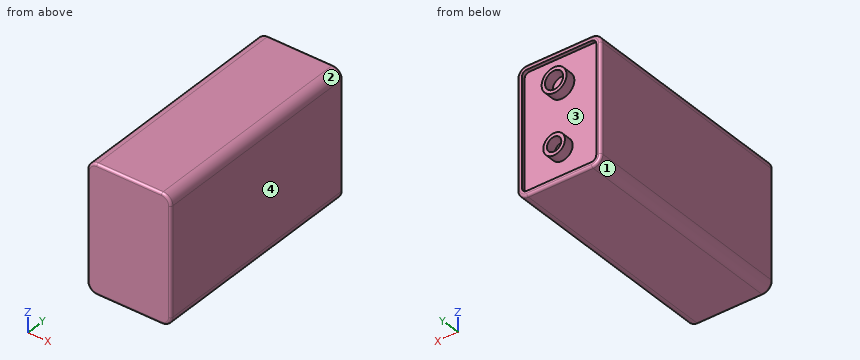
Autodesk Fusion 360 part; units mm, degrees
sketch "Sketch1" plane through (0, 0, 0) normal (0, 1, 0) x (1, 0, 0)
  line L0 (6.75, 13.25) -> (-6.75, 13.25)
  line L1 (-8.75, 11.25) -> (-8.75, -11.25)
  line L2 (-6.75, -13.25) -> (6.75, -13.25)
  line L3 (8.75, -11.25) -> (8.75, 11.25)
  arc A0 (-6.75, 13.25) -> (-8.75, 11.25) centre (-6.75, 11.25) ccw
  arc A1 (8.75, 11.25) -> (6.75, 13.25) centre (6.75, 11.25) ccw
  arc A2 (6.75, -13.25) -> (8.75, -11.25) centre (6.75, -11.25) ccw
  arc A3 (-8.75, -11.25) -> (-6.75, -13.25) centre (-6.75, -11.25) ccw
  point P0 (8.75, 13.25)
  point P1 (-8.75, 13.25)
  point P2 (8.75, -13.25)
  dimension "d1" = 17.5
  dimension "d2" = 26.5
  dimension "d3" = 2
extrude "Extrude1" add sketch "Sketch1" along normal blind 46.4
sketch "Sketch2" plane through (0, 46.4, 0) normal (0, 1, 0) x (-1, 0, 0)
  arc A0 (8.75, 11.25) -> (6.75, 13.25) centre (6.75, 11.25) ccw
  line L0 (6.75, 13.25) -> (-6.75, 13.25)
  arc A1 (-6.75, 13.25) -> (-8.75, 11.25) centre (-6.75, 11.25) ccw
  line L1 (-8.75, 11.25) -> (-8.75, -11.25)
  arc A2 (-8.75, -11.25) -> (-6.75, -13.25) centre (-6.75, -11.25) ccw
  line L2 (-6.75, -13.25) -> (6.75, -13.25)
  arc A3 (6.75, -13.25) -> (8.75, -11.25) centre (6.75, -11.25) ccw
  line L3 (8.75, -11.25) -> (8.75, 11.25)
  line L4 (7.75, -11.25) -> (7.75, 11.25)
  arc A4 (7.75, 11.25) -> (6.75, 12.25) centre (6.75, 11.25) ccw
  line L5 (6.75, 12.25) -> (-6.75, 12.25)
  arc A5 (-6.75, 12.25) -> (-7.75, 11.25) centre (-6.75, 11.25) ccw
  line L6 (-7.75, 11.25) -> (-7.75, -11.25)
  arc A6 (-7.75, -11.25) -> (-6.75, -12.25) centre (-6.75, -11.25) ccw
  line L7 (-6.75, -12.25) -> (6.75, -12.25)
  arc A7 (6.75, -12.25) -> (7.75, -11.25) centre (6.75, -11.25) ccw
  dimension "d6" = -1
extrude "Extrude2" cut sketch "Sketch2" against normal blind 0.75 contours L4 A4 L5 A5 L6 A6 L7 A7
fillet "Fillet1" radius 0.5 16 edges at (0, 46.4, -13.25) (-8.1642, 46.4, -12.6642) (-8.75, 46.4, 0) (-8.1642, 46.4, 12.6642) (0, 46.4, 13.25) (8.1642, 46.4, 12.6642) (8.75, 46.4, 0) (8.1642, 46.4, -12.6642) (0, 0, -13.25) (-8.1642, 0, -12.6642) (-8.75, 0, 0) (-8.1642, 0, 12.6642) (0, 0, 13.25) (8.1642, 0, 12.6642) (8.75, 0, 0) (8.1642, 0, -12.6642)
sketch "Sketch3" plane through (0, 45.65, 0) normal (0, 1, 0) x (-1, 0, 0)
  arc A0 (6.75, -12.25) -> (7.75, -11.25) centre (6.75, -11.25) ccw
  line L0 (7.75, -11.25) -> (7.75, 11.25)
  arc A1 (7.75, 11.25) -> (6.75, 12.25) centre (6.75, 11.25) ccw
  line L1 (6.75, 12.25) -> (-6.75, 12.25)
  arc A2 (-6.75, 12.25) -> (-7.75, 11.25) centre (-6.75, 11.25) ccw
  line L2 (-7.75, 11.25) -> (-7.75, -11.25)
  arc A3 (-7.75, -11.25) -> (-6.75, -12.25) centre (-6.75, -11.25) ccw
  line L3 (-6.75, -12.25) -> (6.75, -12.25)
  circle A4 centre (0, -6.475) radius 2.25
  circle A5 centre (0, 6.475) radius 2.6
  circle A6 centre (0, -6.475) radius 1.5
  circle A7 centre (0, 6.475) radius 1.9
  dimension "d11" = 6.475
  dimension "d12" = 6.475
  dimension "d13" = 4.5
  dimension "d14" = 5.2
  dimension "d15" = -0.75
  dimension "d16" = -0.7
extrude "Extrude3" add sketch "Sketch3" along normal blind 2.1 contours A4 | A5
equation "d11 = ( 12.95 / 2 ) * 1 mm"
equation "d12 = ( 12.95 / 2 ) * 1 mm"
The listing builds one solid part. Answer for the finished solid, in the listing's coordinates (mm). Face numbers are marked on the shaded views. Give positions to 0.01 mm unless a question says otherwise; leave off trailing zeros. Order: outer loops, then holes, each group sorted by start corner. A loop starts at its lowest first (then second) coordinate and runs counter-clockwise, first axis right, second up. Notation, with made-up numbers: (-27, 32.5) - (-22, 32.5) arc R10 cw to (-22, 50.5) - close; hole circle Ø11 at (-14, 44.5). An arc over 180 degrees is marked (long way). Answer as CSV lines item,"result".
Q1. Each of these flat-tipped pins is pushed along its axis until it touches: pin 1 Ø1.1 at (x, z) = (0, 6.5) entering from +Y; pin 2 Ø0.8 at (y, z) = (46, 3.5) entering from +X. Where does it stop, or does it pass through?
Answer key:
pin 1,"stops at y = 45.65"
pin 2,"stops at x = 8.75"
Q2. A cutting plane is placed at C-C, the plane x = 4.75. Determine the outline of the cut face in (y, z), and give its area (3 significant figures).
Answer key:
outline,"(0, -12.75) arc R0.5 ccw to (0.5, -13.25) - (45.9, -13.25) arc R0.5 ccw to (46.4, -12.75) - (46.4, -12.25) - (45.65, -12.25) - (45.65, 12.25) - (46.4, 12.25) - (46.4, 12.75) arc R0.5 ccw to (45.9, 13.25) - (0.5, 13.25) arc R0.5 ccw to (0, 12.75) - close"
area,"1,210 mm^2"
Q3. Straight lines are drawn through the part: L1, parallel to Z at x = 0, y = 46.75 (3 decimals); L2, parallel to Y at x = -4, z = -12; L3, parallel to Y at x = -8, z = 6.5. For each, find the intervals that lie inside material, in ascending order.
Answer key:
L1,"z = -8.725 to -7.975, -4.975 to -4.225, 3.875 to 4.575, 8.375 to 9.075"
L2,"y = 0 to 45.65"
L3,"y = 0 to 46.4"
Q4. A cutting plane is placed at D-D, the plane z = 7. Determine the outline of the cut face in (x, y).
Answer key:
outline,"(-8.75, 0.5) arc R0.5 ccw to (-8.25, 0) - (8.25, 0) arc R0.5 ccw to (8.75, 0.5) - (8.75, 45.9) arc R0.5 ccw to (8.25, 46.4) - (7.75, 46.4) - (7.75, 45.65) - (2.55, 45.65) - (2.55, 47.75) - (1.83, 47.75) - (1.83, 45.65) - (-1.83, 45.65) - (-1.83, 47.75) - (-2.55, 47.75) - (-2.55, 45.65) - (-7.75, 45.65) - (-7.75, 46.4) - (-8.25, 46.4) arc R0.5 ccw to (-8.75, 45.9) - close"
Q5. A cutting plane is placed at A-A, the plane z = -10.5. Determine the outline of the cut face in (x, y).
Answer key:
outline,"(-8.75, 0.5) arc R0.5 ccw to (-8.25, 0) - (8.25, 0) arc R0.5 ccw to (8.75, 0.5) - (8.75, 45.9) arc R0.5 ccw to (8.25, 46.4) - (7.75, 46.4) - (7.75, 45.65) - (-7.75, 45.65) - (-7.75, 46.4) - (-8.25, 46.4) arc R0.5 ccw to (-8.75, 45.9) - close"
Q6. Determine the mould class of the marked faces 1, 2, 3 and 4 for opening direction Z: pulls with the +Z half, pulls with the -Z half, needs draft (parallel to the pull), parting line crosses it, or undercut.
Answer key:
face 1,"pulls with the -Z half"
face 2,"pulls with the +Z half"
face 3,"undercut"
face 4,"needs draft"
Q7. A cutting plane is placed at B-B, the plane x = 0. Determine the outline of the cut face in (y, z) (3 decimals).
Answer key:
outline,"(0, -12.75) arc R0.5 ccw to (0.5, -13.25) - (45.9, -13.25) arc R0.5 ccw to (46.4, -12.75) - (46.4, -12.25) - (45.65, -12.25) - (45.65, -8.725) - (47.75, -8.725) - (47.75, -7.975) - (45.65, -7.975) - (45.65, -4.975) - (47.75, -4.975) - (47.75, -4.225) - (45.65, -4.225) - (45.65, 3.875) - (47.75, 3.875) - (47.75, 4.575) - (45.65, 4.575) - (45.65, 8.375) - (47.75, 8.375) - (47.75, 9.075) - (45.65, 9.075) - (45.65, 12.25) - (46.4, 12.25) - (46.4, 12.75) arc R0.5 ccw to (45.9, 13.25) - (0.5, 13.25) arc R0.5 ccw to (0, 12.75) - close"
